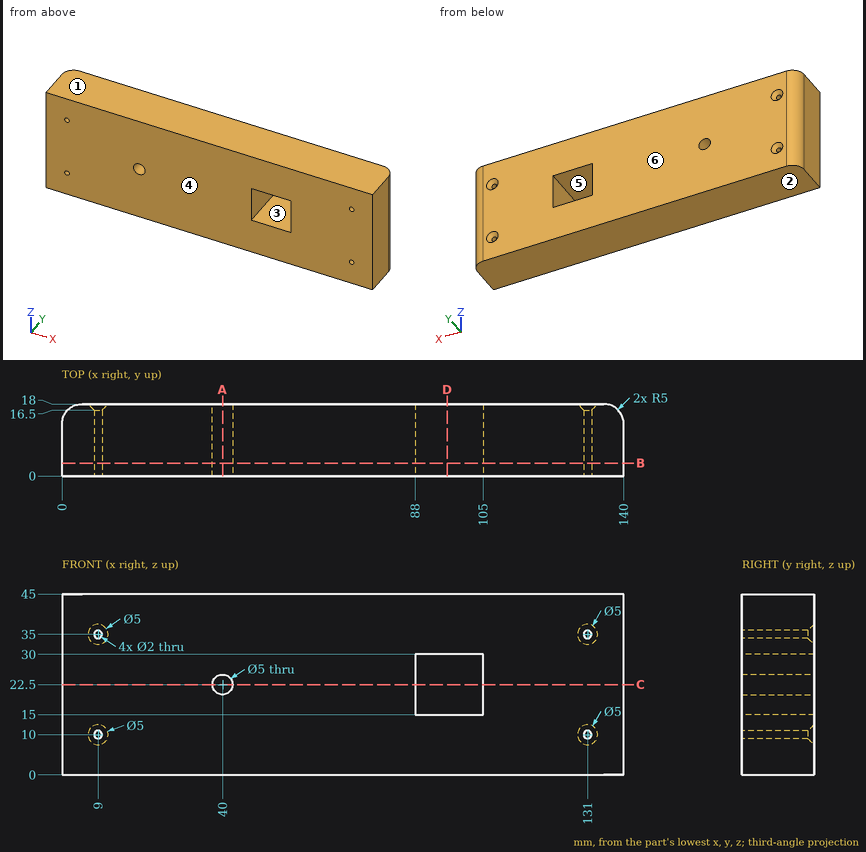
Source: three-view drawing plus pictorial views. Frame: mm from the lowest corner of the part. A direction names the side the tool comes from. Give positions to 0.01 mm unless a question says otherwise; leave off trailing zeros. Order: outer loops, then holes, each group sorted by start corner. A loop starts at its lowest first (then second) coordinate and runs counter-clockwise, first axis right, second up. Notation, with made-up numbers: (85, 83) - (120, 83) arc R14 cw to (120, 105) - close; hole circle Ø10 at (11.5, 83). An arc over 180 degrees is marked (long way). Put each result on its own line as item: value.
Item 1: Access query for the marked faces 5 and 6. Directions: +Z, -Z, +X, -X, +Y, -Y. A direction counts if a zero-diameter tool reaches every point of the face in a straight line with its end or side. Return the directions, or none.
Found:
face 5: +Y, -Y
face 6: +Z, -Z, +X, -X, +Y
Item 2: Section query B-B, the plane y = 3.25. Return loops of the section in (x, z), then the cut area to 3 significant figures.
Found:
outline: (0, 0) - (140, 0) - (140, 45) - (0, 45) - close; hole circle Ø2 at (9, 10); hole circle Ø2 at (9, 35); hole circle Ø5 at (40, 22.5); hole (88, 15) - (105, 15) - (105, 30) - (88, 30) - close; hole circle Ø2 at (131, 10); hole circle Ø2 at (131, 35)
area: 6,010 mm^2
Item 3: Section query D-D, the plane x = 96. Return loops of the section in (y, z), then the cut area to 3 significant figures.
Found:
outline: (0, 0) - (18, 0) - (18, 15) - (0, 15) - close; (0, 30) - (18, 30) - (18, 45) - (0, 45) - close
area: 540 mm^2
Item 4: Section query C-C, the plane z = 22.5. Return loops of the section in (x, y), then the cut area to 3 significant figures.
Found:
outline: (0, 0) - (37.5, 0) - (37.5, 18) - (5, 18) arc R5 ccw to (0, 13) - close; (42.5, 0) - (88, 0) - (88, 18) - (42.5, 18) - close; (105, 0) - (140, 0) - (140, 13) arc R5 ccw to (135, 18) - (105, 18) - close
area: 2,110 mm^2
Item 5: Draft query along Z for the marked faces 1, 2, 3 and 4. Return one class per face: +Z half, -Z half, draft (parallel to the pull), parting line (faces both ways), or undercut.
Found:
face 1: +Z half
face 2: -Z half
face 3: undercut
face 4: draft
Item 6: Contact query for flat-ended pins moving along their axis: pin 1 (2.5 mm diameter, centred on x = 131, z = 35, fed in from +Y); pin 2 (3 mm diameter, centred on x = 9, z = 35, fed in from +Y). Output: stop coordinate, or through.
Found:
pin 1: stops at y = 16.75
pin 2: stops at y = 17
Item 7: Section query A-A, the plane x = 40. Return loops of the section in (y, z).
Found:
outline: (0, 0) - (18, 0) - (18, 20) - (0, 20) - close; (0, 25) - (18, 25) - (18, 45) - (0, 45) - close
Item 8: Ray query, L1, parallel to Z at x = 9, y = 7.75; L2, parallel to X at y = 6.25, z = 10; L3, parallel to X at y = 10.25, z = 22.5. Return the intervals inside material, ascending. Write a range as from..to.
Found:
L1: z = 0..9, 11..34, 36..45
L2: x = 0..8, 10..130, 132..140
L3: x = 0..37.5, 42.5..88, 105..140
